```python
from build123d import *

# Parameters (mm, degrees)
SKETCH_1_W          = 115
SKETCH_1_H          = 90
SKETCH_1_W_2        = 112
SKETCH_1_H_2        = 87
EXTRUDE_1_DEPTH     = 35
SKETCH_3_W          = 115
SKETCH_3_H          = 90
EXTRUDE_2_DEPTH     = 2
SKETCH_4_W          = 20
SKETCH_4_H          = 10
EXTRUDE_3_DEPTH     = 33
FILLET_1_R          = 4
FILLET_2_R          = 4
SKETCH_6_R          = 2.5
CUT_EXTRUDE_1_DEPTH = 33
SKETCH_7_R          = 2.05
CUT_EXTRUDE_2_DEPTH = 170
SKETCH_8_R          = 7.986327153
SKETCH_8_R_2        = 7.617959365
CUT_EXTRUDE_3_DEPTH = 112


with BuildPart() as part:
    # Эскиз1 → Бобышка-Вытянуть1 (new body)
    with BuildSketch(Plane(origin=(0, 0, 0), x_dir=(1, 0, 0), z_dir=(0, 1, 0))):
        with Locations((-57.5, 45)):
            Rectangle(SKETCH_1_W, SKETCH_1_H)
        with Locations((-57.5, 45)):
            Rectangle(SKETCH_1_W_2, SKETCH_1_H_2, mode=Mode.SUBTRACT)
    extrude(amount=EXTRUDE_1_DEPTH)

    # Эскиз3 → Бобышка-Вытянуть2 (add)
    with BuildSketch(Plane(origin=(0, 35, 0), x_dir=(1, 0, 0), z_dir=(0, 1, 0))):
        with Locations((-57.5, 45)):
            Rectangle(SKETCH_3_W, SKETCH_3_H)
    extrude(amount=-EXTRUDE_2_DEPTH)

    # Эскиз4 → Бобышка-Вытянуть3 (add)
    with BuildSketch(Plane.XZ.offset(-33)):
        with Locations((-103.5, -6.5)):
            Rectangle(SKETCH_4_W, SKETCH_4_H)
        with Locations((-103.5, -83.5)):
            Rectangle(SKETCH_4_W, SKETCH_4_H)
        with Locations((-11.5, -83.5)):
            Rectangle(SKETCH_4_W, SKETCH_4_H)
        with Locations((-11.5, -6.5)):
            Rectangle(SKETCH_4_W, SKETCH_4_H)
    extrude(amount=EXTRUDE_3_DEPTH)

    # Скругление1
    fillet_1_edges = [part.edges().sort_by_distance(p)[0] for p in [
        (-113.5, 16.5, -11.5),
        (-93.5, 16.5, -11.5),
        (-93.5, 16.5, -1.5),
        (-113.5, 16.5, -78.5),
        (-93.5, 16.5, -88.5),
        (-93.5, 16.5, -78.5),
        (-1.5, 16.5, -78.5),
        (-21.5, 16.5, -78.5),
        (-21.5, 16.5, -88.5),
        (-1.5, 16.5, -11.5),
        (-21.5, 16.5, -1.5),
        (-21.5, 16.5, -11.5),
    ]]
    fillet(fillet_1_edges, radius=FILLET_1_R)

    # Скругление2
    fillet_2_edges = [part.edges().sort_by_distance(p)[0] for p in [
        (0, 17.5, 0),
        (-115, 17.5, 0),
        (-115, 17.5, -90),
        (0, 17.5, -90),
    ]]
    fillet(fillet_2_edges, radius=FILLET_2_R)

    # Эскиз6 → Вырез-Вытянуть1 (cut)
    with BuildSketch(Plane.XZ):
        with Locations(Location((-107.912454991, -5.546774355, 0), (0, 0, 270))):
            Circle(SKETCH_6_R)
        with Locations(Location((-7.087545009, -84.453225645, 0), (0, 0, 270))):
            Circle(SKETCH_6_R)
        with Locations(Location((-107.912454991, -84.453225645, 0), (0, 0, 270))):
            Circle(SKETCH_6_R)
        with Locations(Location((-7.087545009, -5.546774355, 0), (0, 0, 270))):
            Circle(SKETCH_6_R)
    extrude(amount=-CUT_EXTRUDE_1_DEPTH, mode=Mode.SUBTRACT)

    # Эскиз7 → Вырез-Вытянуть2 (cut)
    with BuildSketch(Plane.ZY.offset(115)):
        with Locations((-45, 17.5)):
            Circle(SKETCH_7_R)
    extrude(amount=-CUT_EXTRUDE_2_DEPTH, mode=Mode.SUBTRACT)

    # Эскиз8 → Вырез-Вытянуть3 (cut)
    with BuildSketch(Plane(origin=(0, 0, -90), x_dir=(-1, 0, 0), z_dir=(0, 0, -1))):
        with Locations((43.5, 17.5)):
            Circle(SKETCH_8_R)
        with Locations((71.5, 17.5)):
            Circle(SKETCH_8_R_2)
    extrude(amount=-CUT_EXTRUDE_3_DEPTH, mode=Mode.SUBTRACT)


solid = part.part
```
Verification items for the finished model (mm, model axes). A direction names the side the tool comes from. Coordinates: 2 decimals unless noted, no trailing zeros. Order: outer loops, then holes, each group sorted by start corner. A loop starts at its lowest first (then second) coordinate and runs counter-clockwise, first axis right, second up. Notation, with made-up numbers: (58, 76) - (65, 76) arc R29 ccw to (65, 113) - close; hole circle Ø4 at (57, 56.25). An arc over 180 degrees is marked (long way). Return JSON: item names as keys, results as strings.
(1) Access from +Z, -Z, +X, -X, +Y, -Y to the whole of each face (thin tool, end or side, straight path). Record for faces 1 (the cylindrical face through (-78.537, 14.582, -0.76)), 2 (the flat face through (-1.5, 13, -45)).
Filled sheet:
{"face 1": "+Z, -Z", "face 2": "-Y"}
(2) Section check D-D, the plane z = -29.5. Record the cut outline in (x, y), and give its area (3 significant figures).
Filled sheet:
{"outline": "(-115, 0) - (-113.5, 0) - (-113.5, 33) - (-1.5, 33) - (-1.5, 0) - (0, 0) - (0, 35) - (-115, 35) - close", "area": "329 mm^2"}
(3) Thickness scan on line 1 along Z through (x, y) = (-108, 30.5); line 2 along Z through (x, y) = (-85, 18); line 3 along X through (y, z) = (26, -40.5). Record the ranges inside material, lowest first.
Filled sheet:
{"line 1": "z = -90 to -86.95, -81.95 to -78.5, -11.5 to -8.05, -3.05 to 0", "line 2": "z = -90 to -88.5, -1.5 to 0", "line 3": "x = -115 to -113.5, -1.5 to 0"}
(4) Section check C-C, the plane x = -32. Record the cut outline in (y, z).
Filled sheet:
{"outline": "(0, -90) - (35, -90) - (35, 0) - (0, 0) - (0, -1.5) - (33, -1.5) - (33, -88.5) - (0, -88.5) - close"}
(5) Go/stop test with a flat-tipped pin: pin 1 (8 mm diameter, centred on x = -21.5, z = -63.5, fed in from -Y). Record where the tip stops, or that it passes through.
Filled sheet:
{"pin 1": "stops at y = 33"}
(6) Section check B-B, the plane z = -44.5. Record the cut outline in (x, y), and give its area (3 significant figures).
Filled sheet:
{"outline": "(-115, 0) - (-113.5, 0) - (-113.5, 15.51) - (-115, 15.51) - close; (-115, 19.49) - (-113.5, 19.49) - (-113.5, 33) - (-1.5, 33) - (-1.5, 19.49) - (0, 19.49) - (0, 35) - (-115, 35) - close; (-1.5, 0) - (0, 0) - (0, 15.51) - (-1.5, 15.51) - close", "area": "317 mm^2"}
(7) Section check A-A, the plane x = -43.5. Record the cut outline in (y, z).
Filled sheet:
{"outline": "(0, -90) - (9.51, -90) - (9.51, -88.5) - (0, -88.5) - close; (0, -1.5) - (9.51, -1.5) - (9.51, 0) - (0, 0) - close; (25.49, -90) - (35, -90) - (35, 0) - (25.49, 0) - (25.49, -1.5) - (33, -1.5) - (33, -88.5) - (25.49, -88.5) - close"}
(8) Mould release check, pull along Z, two halves, no side actions. Record for faces 3 (the flat face through (-58, 0, -1)), 4 (the cylindrical face through (-92.359, 16.269, -2.703)): pulls with the +Z half, pulls with the -Z half, needs draft (parallel to the pull), parting line crosses it, or undercut.
Filled sheet:
{"face 3": "needs draft", "face 4": "undercut"}
